Autodesk Inventor part; units mm, degrees
ref_plane "Work Plane1" through (-1107.6248, 3927.9173, 0) normal (0, 0, 1) x (-0.9927008, 0.1206028, 0)
ref_plane "Work Plane7" through (-17.5791, -32.927, 3.4) normal (0, 0, -1) x (0.0194385, 0.9998111, 0)
ref_plane "Work Plane8" through (-22.6017, 2.8462, 4) normal (0, 0, -1) x (0.4990785, 0.8665568, 0)
ref_plane "Work Plane1" through (-1107.6248, 3927.9173, 0) normal (0, 0, 1) x (-0.9927008, 0.1206028, 0)
sketch "Sketch1" plane through (-1107.6248, 3927.9173, 0) normal (0, 0, 1) x (-0.9927008, 0.1206028, 0)
  circle A0 centre (14.5, -14.5) radius 13.85
  circle A1 centre (14.5, -14.5) radius 14.5
  circle A2 centre (14.5, -55.2958) radius 13.85
  circle A3 centre (14.5, -55.2958) radius 14.5
  circle A4 centre (13, -35.0012) radius 5
  line L0 (0, 0) -> (29, 0)
  line L1 (29, 0) -> (29, -67)
  line L2 (29, -67) -> (0, -67)
  line L3 (0, -67) -> (0, 0)
  line L4 (2, 0) -> (2, -67)
  line L5 (14.5, -28.35) -> (2, -28.35)
  line L6 (14.5, -29) -> (2, -29)
  line L7 (14.5, -40.7958) -> (2, -40.7958)
  line L8 (14.5, -41.4458) -> (2, -41.4458)
  line L9 (19, 0) -> (19, -67)
  point P0 (-1573.2578, 3765.6642)
  point P1 (19, -42.1973)
  point P2 (19, -27.5986)
  point P3 (19, -41.5118)
  point P4 (19, -28.284)
  dimension "d0" = 67
  dimension "d1" = 2
  dimension "d2" = 1
ref_plane "Work Plane7" through (-17.5791, -32.927, 3.4) normal (0, 0, -1) x (0.0194385, 0.9998111, 0)
extrude "Extrusion1" add sketch "Sketch1" along normal blind 3.8 contours L9 A1 L5 A0 | L9 A3 L7 L4 L6 A1 | A1 L6 L4 L5 | L9 A2 L8 A3 | A3 L8 L4 L7
ref_plane "Work Plane8" through (-22.6017, 2.8462, 4) normal (0, 0, -1) x (0.4990785, 0.8665568, 0)
ref_plane "Work Plane9" through (151.4324, -161.9595, 4) normal (0, 0, 1) x (0.0950598, 0.9954716, 0)
sketch "Sketch2" plane through (-1107.6248, 3927.9173, 3.8) normal (0, 0, 1) x (0.9927008, -0.1206028, 0)
  arc A0 (-19, 42.1973) -> (-14.5, 41.4458) centre (-14.5, 55.2958) ccw
  line L0 (-19, 42.1973) -> (-19, 27.5986)
  arc A1 (-14.5, 28.35) -> (-19, 27.5986) centre (-14.5, 14.5) ccw
  line L1 (-14.5, 28.35) -> (-2, 28.35)
  line L2 (-2, 28.35) -> (-2, 41.4458)
  line L3 (-2, 41.4458) -> (-14.5, 41.4458)
  circle A2 centre (-13, 35.0012) radius 5
  circle A3 centre (-20.1246, 52.8194) radius 14.7
  line L4 (-20.1246, 38.1194) -> (-2, 38.1194)
  line L5 (-2, 28.35) -> (-2, 41.4458)
  line L6 (-20.1246, 52.8194) -> (-20.1246, 38.1194)
  point P0 (-2, 38.1194)
  point P1 (-19, 38.1625)
  point P2 (-10.8116, 41.4458)
  point P3 (-19, 38.1194)
extrude "Extrusion4" add sketch "Sketch2" along normal blind 0.4
sketch "Sketch3" plane through (-1106.1911, 3956.3016, 0) normal (0.9927008, -0.1206028, 0) x (0, 0, -1)
  line L0 (0, 0) -> (-4.2, 0)
  line L1 (0, 0) -> (0, 13.0958)
  line L2 (0, 13.0958) -> (-4.2, 13.0958)
  line L3 (-4.2, 6.5479) -> (0, 6.5479)
  line L4 (-4.2, 6.5479) -> (0, 0)
  line L5 (-4.2, 6.5479) -> (0, 13.0958)
  line L6 (0, 6.5479) -> (-2.1, 9.8219)
  line L7 (0, 6.5479) -> (-2.1, 3.274)
  line L8 (-4.2, 0) -> (-4.2, 13.0958)
  point P0 (0, -3794.0142)
  dimension "d11" = 6.5479
  dimension "d12" = 6.5479
hole "Hole1" at (-1105.7963, 3959.5516, 2.1) at (-1105.0066, 3966.0518, 2.1) direction (-0.9927008, 0.1206028, 0) diameter 3.5 depth 4.5 counterbore diameter 4 counterbore depth 0.5
equation "\"d11\" = d12"
properties part number "BearigHold"
Can you work these out from the model? Positions are in its coordinate system, mm. A direction names the side the tool comes from. Coordinates: 2 decimals unless noted, no trailing zeros. Write each loop counter-clockwise with the first axis right and the second up, starting at its lowest first coordinate (ties: lowest second). Pieces come first, ordered by that corner, then holes. Notation, with made-up numbers: (39.5, 86) - (85.5, 86) arc R9 cw to (85.5, 90) - close; hole circle Ø3 at (4, 30.25). An arc over 180 degrees is marked (long way). Return JSON: item names as keys, results as strings.
Q1. If we section it at C-C (x = -1120.5): Please give me the cut outline in (y, z).
Computed values:
{"outline": "(3957.91, 0) - (3961.5, 0) - (3961.5, 3.8) - (3966.96, 3.8) - (3966.96, 0) - (3971.7, 0) - (3971.7, 3.8) - (3997.46, 3.8) - (3997.46, 4.2) - (3957.91, 4.2) - close"}
Q2. I'm going to push flat-ended pins straight in: pin 1 Ø1.5 at (x, y) = (-1127.5, 3980.5) entering from -Z; pin 2 Ø2 at (y, z) = (3981, 3.5) entering from -X. Where does each tip first touch, or does it pass through?
Computed values:
{"pin 1": "stops at z = 3.8", "pin 2": "stops at x = -1135.91"}
Q3. Please list where these lines run through material, in increasing order: L1, parallel to Z at x = -1113, y = 3989.5; L2, parallel to Y at x = -1112, z = 2.35; L3, parallel to Y at x = -1107, z = 1.6. Write a range as from..to.
Computed values:
{"L1": "z = 3.8..4.2", "L2": "y = 3957.01..3961.69, 3966.77..3970.2", "L3": "y = 3956.4..3958.01, 3961.39..3964.6, 3967.98..3969.59"}
Q4. If we section it at D-D (y = 3975): Please give me the cut outline in (x, z).
Computed values:
{"outline": "(-1133.71, 3.8) - (-1108.76, 3.8) - (-1108.76, 4.2) - (-1133.71, 4.2) - close"}
Q5. If we section it at A-A (z = 2.4): Please give me the cut outline in (x, y).
Computed values:
{"outline": "(-1123.16, 3957.61) arc R13.85 cw to (-1118.6, 3957.81) - (-1106.19, 3956.3) - (-1106.03, 3957.59) - (-1106.53, 3957.65) - (-1106.5, 3957.9) - (-1110.47, 3958.38) - (-1110.06, 3961.81) - (-1106.08, 3961.32) - (-1106.05, 3961.57) - (-1105.56, 3961.51) - (-1105.25, 3964.09) - (-1105.74, 3964.15) - (-1105.71, 3964.4) - (-1109.68, 3964.88) - (-1109.27, 3968.31) - (-1105.3, 3967.82) - (-1105.26, 3968.08) - (-1104.77, 3968.01) - (-1104.61, 3969.3) - (-1117.02, 3970.81) arc R13.85 cw to (-1121.4, 3972.1) - close; hole circle Ø10 at (-1116.31, 3964.23)"}
Q6. On a 3-axis mill with a long thin cutter (end or side, diameter ignored), from which of +Z, -Z, +X, -X, +Y, -Y can I reach the whole of each face in a straight line? I mean faces 1 (the cylindrical face through (-1119.231, 3971.263, 1.873)), 2 (the flat face through (-1110.266, 3960.07, 2.124)), 3 (the flat face through (-1116, 3964, 3.8)), 4 (the cylindrical face through (-1120.919, 3957.895, 1.873)), 5 (the flat face through (-1111, 3967, 0)). Say none if no direction works.
Computed values:
{"face 1": "-Z, +X, +Y", "face 2": "none", "face 3": "-Z", "face 4": "+Z, -Z, -Y", "face 5": "-Z, +X, -X, +Y, -Y"}
Q7. Thinking about a two-plate mould opening in X: for faces 6 (the cylindrical face through (-1112.74, 3960.73, 1.87)), 7 (the flat face through (-1110.903, 3970.066, 2.071)), 8 (the flat face through (-1120, 3978, 4.2)), which applies, +X half, -X half, draft (parallel to the pull), parting line (faces both ways), or undercut?
Computed values:
{"face 6": "undercut", "face 7": "+X half", "face 8": "draft"}
Q8. If we section it at B-B (x = -1112.5): Please give me the cut outline in (y, z).
Computed values:
{"outline": "(3957.07, 0) - (3960.99, 0) - (3960.99, 3.8) - (3967.47, 3.8) - (3967.47, 0) - (3970.26, 0) - (3970.26, 4.2) - (3957.07, 4.2) - close; (3970.95, 3.8) - (3994.6, 3.8) - (3994.6, 4.2) - (3970.95, 4.2) - close"}
